```python
from build123d import *

# Parameters (mm, degrees)
F0_W     = 910
F0_H     = 1730
F1_DEPTH = 890
F2_W     = 1400
F2_H     = 380
F3_DEPTH = 610
F4_W     = 165
F4_H     = 190
F5_DEPTH = 610


with BuildPart() as f1:
    # F0 (on Top) → F1 (new body)
    with BuildSketch(Plane.XY):
        with Locations((10.50148, 0)):
            Rectangle(F0_W, F0_H)
    extrude(amount=F1_DEPTH)

    # F2 (on face) → F3 (cut)
    with BuildSketch(Plane(origin=(-444.49852, 0, 0), x_dir=(0, -1, 0), z_dir=(-1, 0, 0))):
        with Locations((0, 700)):
            Rectangle(F2_W, F2_H)
    extrude(amount=-F3_DEPTH, mode=Mode.SUBTRACT)

    # F4 (on face) → F5 (cut, through all)
    with BuildSketch(Plane(origin=(-444.49852, 0, 0), x_dir=(0, -1, 0), z_dir=(-1, 0, 0))):
        with Locations((-782.5, 795)):
            Rectangle(F4_W, F4_H)
        with Locations((782.5, 795)):
            Rectangle(F4_W, F4_H)
    extrude(amount=-F5_DEPTH, mode=Mode.SUBTRACT)


solid = f1.part
```
For this review, take the finished solid that the model builds, in its own axes (mm). A direction names the side the tool comes from. Round coordinates to 2 decimals unless told otherwise and drop trailing zeros. Loops run counter-clockwise (first coordinate to the right, second up) from the corner with the lowest first, then second, coordinate; pieces in that order, holes last.
Q1. Mouldability with a two-part tool opening along Y and no side actions: class faces 1 (the face through (-144, 10, 510)), 2 (the face through (4, -865, 340)), 3 (the face through (313, 12, 890)) as +Y half, -Y half, draft (parallel to the pull), parting line (faces both ways), or undercut.
Result sheet:
face 1: undercut
face 2: -Y half
face 3: draft
Q2. Add section A-A on z = 542.5. Write out the cut boundary in (x, y).
Result sheet:
outline: (-444.5, -865) - (465.5, -865) - (465.5, 865) - (-444.5, 865) - (-444.5, 700) - (165.5, 700) - (165.5, -700) - (-444.5, -700) - close
Q3. Machinability: for faces 4 (the face through (-144, -781, 700)), 5 (the face through (-144, 700, 604)), 6 (the face through (4, 865, 340)), which of the approach directions +Z, -Z, +X, -X, +Y, -Y give a long, thin tool a straight path to every point of the face, cutting with its end or side? Answer none if there is none.
Result sheet:
face 4: +Z, -X, +Y, -Y
face 5: +Z, -X
face 6: +Z, -Z, +X, -X, +Y
Q4. Insertion check: pin 1 Ø5 at (x, y) = (132, -77.5) entering from +Z. The pin has a flat end and moves straight along its axis. Give the tip position at first contact, or say it passes through.
Result sheet:
pin 1: stops at z = 510
Q5. Add section D-D on z = 757. Write out the cut boundary in (x, y), plus the area to 3 significant figures.
Result sheet:
outline: (165.5, -865) - (465.5, -865) - (465.5, 865) - (165.5, 865) - close
area: 519,000 mm2
Q6. Add section C-C on x = -52.5. Write out the cut boundary in (y, z), plus the area to 3 significant figures.
Result sheet:
outline: (-865, 0) - (865, 0) - (865, 700) - (700, 700) - (700, 510) - (-700, 510) - (-700, 700) - (-865, 700) - close
area: 945,000 mm2
Q7. To check wall thickness, follow line 1 along X through (y, z) = (-721, 796); line 2 along Z through (x, y) = (-310, -775.5); line 3 along Z through (x, y) = (-395, 268.5). State the ranges of each line that lie inside material, in increasing order.
Result sheet:
line 1: x = 165.5 to 465.5
line 2: z = 0 to 700
line 3: z = 0 to 510
Q8. Add section B-B on y = 462.5. Write out the cut boundary in (x, z).
Result sheet:
outline: (-444.5, 0) - (465.5, 0) - (465.5, 890) - (165.5, 890) - (165.5, 510) - (-444.5, 510) - close
